```python
from build123d import *

# Parameters (mm, degrees)
SKETCH1_W           = 152.4
SKETCH1_H           = 76.2
BOSS_EXTRUDE1_DEPTH = 3.175
CUT_EXTRUDE1_DEPTH  = 3.175
FILLET2_R           = 2.54
FILLET3_R           = 2.54
SKETCH5_R           = 7.62
CUT_EXTRUDE2_DEPTH  = 3.175
SKETCH6_R           = 1.27
CUT_EXTRUDE3_DEPTH  = 3.175
BOSS_EXTRUDE2_START = -3.175
SKETCH7_R           = 7.62
SKETCH7_R_2         = 3.25
BOSS_EXTRUDE2_DEPTH = 3.175


with BuildPart() as part:
    # Sketch1 → Boss-Extrude1 (new body)
    with BuildSketch(Plane(origin=(0, 0, 0), x_dir=(1, 0, 0), z_dir=(0, 1, 0))):
        Rectangle(SKETCH1_W, SKETCH1_H)
    extrude(amount=BOSS_EXTRUDE1_DEPTH)

    # Sketch4 → Cut-Extrude1 (cut)
    with BuildSketch(Plane(origin=(0, 3.175, 0), x_dir=(1, 0, 0), z_dir=(0, 1, 0))):
        with BuildLine():
            Line((0, 38.1), (76.2, 38.1))
            Line((76.2, 38.1), (76.2, 12.7))
            ThreePointArc((76.2, 12.7), (40.160926284, 31.582778852), (0, 38.1))
        make_face()
        with BuildLine():
            Line((76.2, -38.1), (76.2, -12.7))
            ThreePointArc((76.2, -12.7), (40.160926284, -31.582778852), (0, -38.1))
            Line((0, -38.1), (76.2, -38.1))
        make_face()
    extrude(amount=-CUT_EXTRUDE1_DEPTH, mode=Mode.SUBTRACT)

    # Fillet2
    fillet2_edges = [part.edges().sort_by_distance(p)[0] for p in [
        (76.2, 1.5875, -12.7),
        (76.2, 1.5875, 12.7),
    ]]
    fillet(fillet2_edges, radius=FILLET2_R)

    # Fillet3
    fillet3_edges = [part.edges().sort_by_distance(p)[0] for p in [
        (-76.2, 1.5875, -38.1),
        (-76.2, 1.5875, 38.1),
    ]]
    fillet(fillet3_edges, radius=FILLET3_R)

    # Sketch5 → Cut-Extrude2 (cut)
    with BuildSketch(Plane(origin=(0, 3.175, 0), x_dir=(1, 0, 0), z_dir=(0, 1, 0))):
        with Locations(Location((50.8, 0, 0), (0, 0, 270))):
            Circle(SKETCH5_R)
    extrude(amount=-CUT_EXTRUDE2_DEPTH, mode=Mode.SUBTRACT)

    # Sketch6 → Cut-Extrude3 (cut)
    with BuildSketch(Plane(origin=(0, 3.175, 0), x_dir=(1, 0, 0), z_dir=(0, 1, 0))):
        with Locations(Location((-63.5, 25.4, 0), (0, 0, 270))):
            Circle(SKETCH6_R)
        with Locations(Location((-63.5, -25.4, 0), (0, 0, 270))):
            Circle(SKETCH6_R)
        with Locations(Location((-24.13, 25.4, 0), (0, 0, 270))):
            Circle(SKETCH6_R)
        with Locations(Location((-24.13, -25.4, 0), (0, 0, 270))):
            Circle(SKETCH6_R)
    extrude(amount=-CUT_EXTRUDE3_DEPTH, mode=Mode.SUBTRACT)

    # Sketch7 → Boss-Extrude2 (add)
    with BuildSketch(Plane.XZ.offset(BOSS_EXTRUDE2_START)):
        with Locations((50.8, 0)):
            Circle(SKETCH7_R)
        with Locations(Location((50.8, 0, 0), (0, 0, 270))):
            Circle(SKETCH7_R_2, mode=Mode.SUBTRACT)
    extrude(amount=BOSS_EXTRUDE2_DEPTH)


solid = part.part
```
Can you work these out from the model? Positions are in its coordinate system, mm. Round coordinates to 2 decimals unless told otherwise and drop trailing zeros. Order: outer loops, then holes, each group sorted by start corner. A loop starts at its lowest first (then second) coordinate and runs counter-clockwise, first axis right, second up.
(1) If we section it at B-B (y = 1.7): Please give me the cut outline in (x, z), plus the area to 3 significant figures.
Results are:
outline: (-76.2, -35.56) arc R2.54 ccw to (-73.66, -38.1) - (0, -38.1) arc R127 ccw to (75.16, -13.47) arc R2.54 ccw to (76.2, -11.42) - (76.2, 11.42) arc R2.54 ccw to (75.16, 13.47) arc R127 ccw to (0, 38.1) - (-73.66, 38.1) arc R2.54 ccw to (-76.2, 35.56) - close; hole circle Ø2.54 at (-63.5, -25.4); hole circle Ø2.54 at (-63.5, 25.4); hole circle Ø2.54 at (-24.13, -25.4); hole circle Ø2.54 at (-24.13, 25.4); hole circle Ø6.5 at (50.8, 0)
area: 10,300 mm2
(2) If we section it at D-D (x = 32.5): Please give me the cut outline in (y, z) (3 decimals), plus the area to 3 significant figures.
Results are:
outline: (0, -33.871) - (3.175, -33.871) - (3.175, 33.871) - (0, 33.871) - close
area: 215 mm2
(3) If I drill on L1, parallel to X at y = 2.25, z = 0; L2, parallel to X at y = 0.2, z = 1; L3, parallel to X at y = 1.35, z = 25.4, over which ranges is the centre line in solid material (lowest first)?
Results are:
L1: x = -76.2 to 47.55, 54.05 to 76.2
L2: x = -76.2 to 47.71, 53.89 to 76.2
L3: x = -76.2 to -64.77, -62.23 to -25.4, -22.86 to 55.36
(4) I'm going to push flat-ended pins straight in: pin 1 (10.5 mm diameter, centred on x = 50.8, z = 0, fed in from +Y) (3 decimals); pin 2 (1.5 mm diameter, centred on y = 0.5, z = -19.5, fed in from +X). Where does each tip first touch, or does it pass through?
Results are:
pin 1: stops at y = 3.175
pin 2: stops at x = 67.38
(5) If we section it at C-C (x = 50.8): Please give me the cut outline in (y, z) (3 decimals).
Results are:
outline: (0, -27.497) - (3.175, -27.497) - (3.175, -3.25) - (0, -3.25) - close; (0, 3.25) - (3.175, 3.25) - (3.175, 27.497) - (0, 27.497) - close
(6) If we section it at A-A (z = 0): Please give me the cut outline in (x, y) (3 decimals), plus the area to 3 significant figures.
Results are:
outline: (-76.2, 0) - (47.55, 0) - (47.55, 3.175) - (-76.2, 3.175) - close; (54.05, 0) - (76.2, 0) - (76.2, 3.175) - (54.05, 3.175) - close
area: 463 mm2
(7) We'd pull the mould along Z, two halves only. Please class faces 1 (the face through (-76.2, 2, 0)), 2 (the face through (40.08, 1.61, -31.61)), 3 (the face through (47.627, 1.61, 0.705)), 4 (the face through (-37, 2, 38.1)): +Z half, -Z half, draft (parallel to the pull), parting line (faces both ways), or undercut.
Results are:
face 1: draft
face 2: -Z half
face 3: undercut
face 4: +Z half
